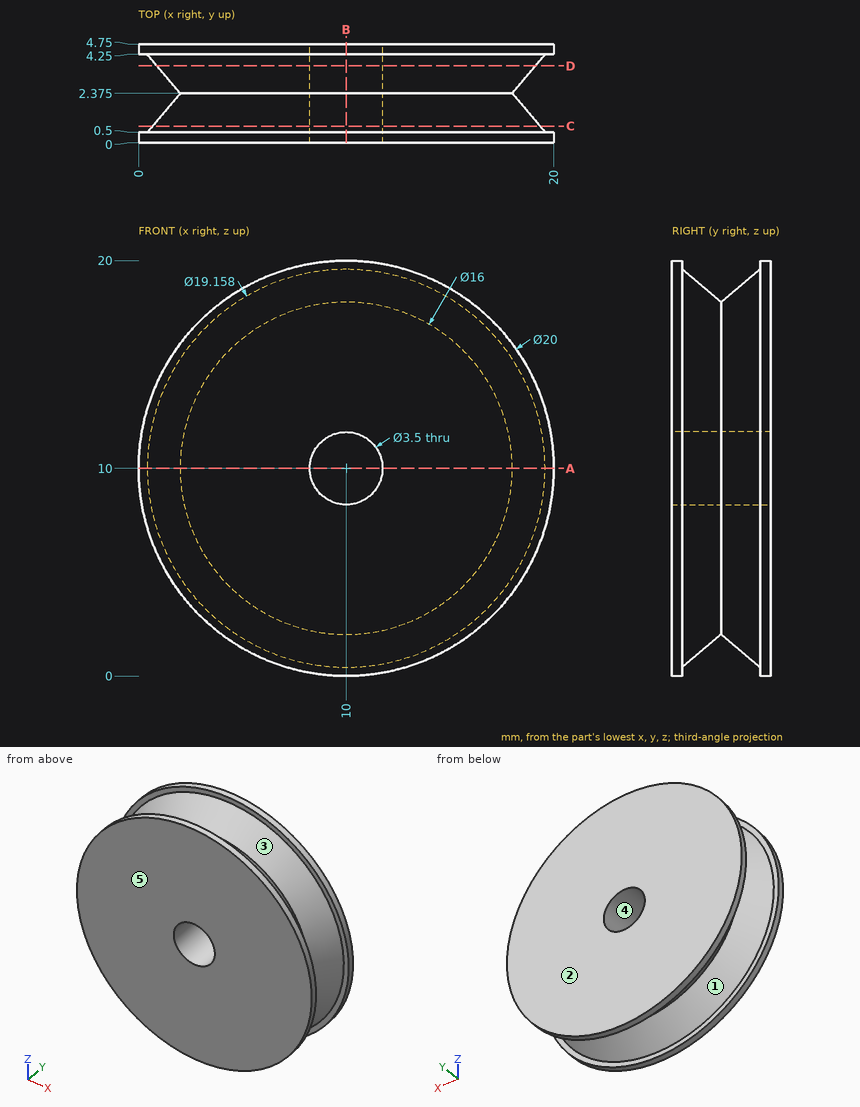
Here's the drawing with two shaded views (mm, measured from the low corner). I have some questions. A direction names the side the tool comes from. Coordinates: 2 decimals unless noted, no trailing zeros. Order: outer loops, then holes, each group sorted by start corner. A loop starts at its lowest first (then second) coordinate and runs counter-clockwise, first axis right, second up. Notation, with made-up numbers: M 6.25,67 L 54.25,67 A12 ccw 54.25,74 Z; hole C 20,-34 d1. An arc over 180 degrees is marked long. Write item = value, one per line.
(1) Suppose I cut it at B-B on x = 10. Please give me the cut outline in (y, z) (3 decimals), plus the area to 3 significant figures.
Results are:
outline = M 0,0 L 0.5,0 L 0.5,0.421 L 2.375,2 L 4.25,0.421 L 4.25,0 L 4.75,0 L 4.75,8.25 L 0,8.25 Z; M 0,11.75 L 4.75,11.75 L 4.75,20 L 4.25,20 L 4.25,19.579 L 2.375,18 L 0.5,19.579 L 0.5,20 L 0,20 Z
area = 69.3 mm2
(2) Suppose I cut it at A-A on z = 10. Please give me the cut outline in (x, y) (3 decimals).
Results are:
outline = M 0,0 L 8.25,0 L 8.25,4.75 L 0,4.75 L 0,4.25 L 0.421,4.25 L 2,2.375 L 0.421,0.5 L 0,0.5 Z; M 11.75,0 L 20,0 L 20,0.5 L 19.579,0.5 L 18,2.375 L 19.579,4.25 L 20,4.25 L 20,4.75 L 11.75,4.75 Z
(3) For pin 1 Ø1 at (y, z) = (2, 2.5) entering from -X; pin 2 Ø4 at (x, z) = (10, 10) entering from -Y; pin 3 Ø1 at (y, z) = (3.5, 18) entering from -X, each with a flat end and sliding along its axis, tell me the tip position at first contact or that it passes through.
Results are:
pin_1 = 5.19
pin_2 = 0
pin_3 = 4.8
(4) For the marked faces 1 and 2, which set-ups out of +Z, -Z, +X, -X, +Y, -Y let a thin tool reach every point of the face, with its end or its side?
Results are:
face_1 = none
face_2 = +Z, -Z, +X, -X, +Y
(5) Suppose I cut it at D-D on y = 3.7. Please give me the cut outline in (x, z), plus the area to 3 significant figures.
Results are:
outline = C 10,10 d18.23; hole C 10,10 d3.5
area = 251 mm2
(6) If we mould it in two halves opening along Y, with no side actions, what happens to the marked faces 3, 4 and 5? For each: pulls with the +Y half, pulls with the -Y half, needs draft (parallel to the pull), parting line crosses it, or undercut.
Results are:
face_3 = undercut
face_4 = needs draft
face_5 = pulls with the -Y half
(7) Suppose I cut it at C-C on y = 0.8. Please give me the cut outline in (x, z).
Results are:
outline = C 10,10 d18.65; hole C 10,10 d3.5
(8) I need wall thicknesses on line 1 along Y through (x, z) = (4, 3); line 2 along X through (y, z) = (2, 10); line 3 along Y through (x, z) = (3.5, 5). Which ranges of each line are inside material? Lowest first, please. Write a range as [from, to].
Results are:
line_1 = [0, 0.93], [3.82, 4.75]
line_2 = [1.68, 8.25], [11.75, 18.32]
line_3 = [0, 2.14], [2.61, 4.75]
